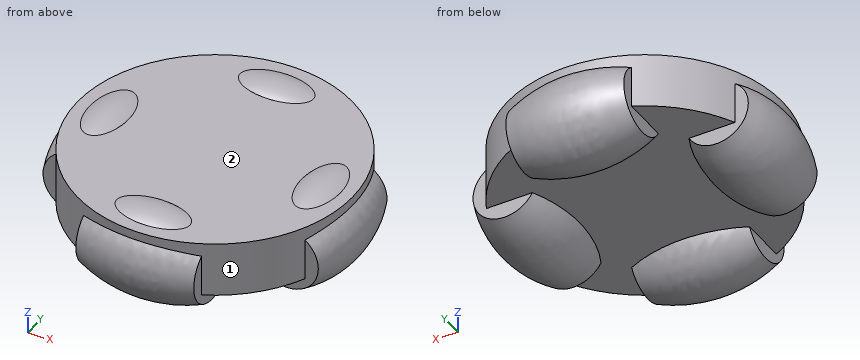
from build123d import *

# Parameters (mm, degrees)
EXTRUDE_1_DEPTH          = 5
EXTRUDE_1_DEPTH_BACK     = 2
SKETCH_2_R               = 17.5
PATTERN_CIRCULAR_1_COUNT = 4


with BuildPart() as part:
    # ｽｹｯﾁ1 → 回転1 (revolve)
    with BuildSketch(Plane.XY, mode=Mode.PRIVATE) as revolve_1_sk:
        with BuildLine():
            Line((-7.5, 17.511496224), (-7.5, 13.470384182))
            Line((-7.5, 13.470384182), (7.5, 13.470384182))
            Line((7.5, 13.470384182), (7.5, 17.511496224))
            ThreePointArc((7.5, 17.511496224), (0, 19.05), (-7.5, 17.511496224))
        make_face()
    revolve_1 = revolve(revolve_1_sk.sketch.rotate(Axis((-13.470384182, 13.470384182, 0), (1, 0, 0)), 90), axis=Axis((-13.470384182, 13.470384182, 0), (1, 0, 0)))

    # ｽｹｯﾁ2 → ﾎﾞｽ - 押し出し1 (add, two sides: drawn at the far end of the back side and taken through both)
    with BuildSketch(Plane.XY.offset(-EXTRUDE_1_DEPTH_BACK)):
        Circle(SKETCH_2_R)
    extrude(amount=EXTRUDE_1_DEPTH + EXTRUDE_1_DEPTH_BACK)

    # 円形ﾊﾟﾀｰﾝ1: 回転1 ×4 about axis
    pattern_circular_1_axis = Axis((0, 0, 0), (0, 0, 1))
    for i in range(1, PATTERN_CIRCULAR_1_COUNT):
        add(revolve_1.rotate(pattern_circular_1_axis, i * 360 / PATTERN_CIRCULAR_1_COUNT))


solid = part.part
For this review, take the finished solid that the model builds, in its own axes (mm). Face numbers are marked on the shaded views. Give positions to 0.01 mm unless a question says otherwise; leave off trailing zeros. Answer in a Markdown table with one row per item. Add a question column.
(1) Mouldability with a two-part tool opening along Y and no side actions: class the marked faces 1 and 2 as +Y half, -Y half, draft (parallel to the pull), parting line (faces both ways), or undercut.
(2) Wall thickness on probe 1 along Z at (x, y) = (3.5, -4); probe 2 along X at (y, z) = (7.5, 4); probe 3 along X at (y, z) = (5, -2.75): over which ranges is each line inside the solid? List them lowest first. Write a range as [from, to].
(3) For pin 1 (3.5 mm diameter, centred on y = 15.5, z = -0.5, fed in from -X); pin 2 (16 mm diameter, centred on x = 2.5, y = 2, fed in from -Z); pin 3 (12 mm diameter, centred on x = -14.5, y = 9, fed in from -Z); pin 4 (8 mm diameter, centred on x = -14, y = 3, fed in from -Z), all flat-tipped, find the tip position at first contact; note any pin that passes through.
Evaluation:
| question | item | result |
|---|---|---|
| 1 | face 1 | parting line |
| 1 | face 2 | undercut |
| 2 | probe 1 | z = [-2, 5] |
| 2 | probe 2 | x = [-15.81, 15.81] |
| 2 | probe 3 | x = [-17.54, -9.4], [9.4, 17.54] |
| 3 | pin 1 | stops at x = -10.83 |
| 3 | pin 2 | stops at z = -4.65 |
| 3 | pin 3 | stops at z = -5.33 |
| 3 | pin 4 | stops at z = -5.58 |
